Check sheet for the drawn part. Datum: minimum x, y, z corner. Units: mm. A direction names the side the tool comes from. Round coordinates to 2 decimals unless told otherwise and drop trailing zeros. Write each loop counter-clockwise with the first axis right and the second up, starting at its lowest first coordinate (ties: lowest second). Pieces come first, ordered by that corner, then holes. Notation, with made-up numbers: (-17, 78) - (-6, 78) arc R20 ccw to (-6, 109) - close; hole circle Ø5 at (-3, 36). An arc over 180 degrees is marked (long way). Answer as a JSON object with one key per item and string values. Group by question number.
Item 1: Sectioned sample at D-D on z = 56.5. Record the boundary of the cut face in (x, y), plus the area to 3 significant figures.
Item 2: Release check for a two-part mould opening along Y. For the marked faces 1, 2, 3 and 4 record: pulls with the +Y half, pulls with the -Y half, needs draft (parallel to the pull), parting line crosses it, or undercut.
Item 3: Thickness scan on line 1 (Z direction, x = 70, y = 37.5); line 2 (Z direction, x = 38, y = 93); line 3 (Y direction, x = 38, z = 20). Record the ranges inside material, lowest first.
Item 4: Sectioned sample at B-B on x = 47. Record the boundary of the cut face in (y, z).
Item 5: Sectioned sample at C-C on y = 93.98. Record the boundary of the cut face in (x, z).
Item 6: Gauge pin test, flat ends, axial feed: P1, Ø12, axis at y = 93.98, z = 20.32, coming from the -X side; P2, Ø8, axis at x = 41.5, y = 31.5, coming from the +Z side; P3, Ø1.5, axis at x = 60.5, y = 121, coming from the -Z side. Record the tip position at first contact, or that the pin passes through.
Item 7: Set-up check for the marked faces 5 and 6: record each of +Z, -Z, +X, -X, +Y, -Y from which the full face is reachable in a straight line by a thin tool's end or side.
Item 8: Sectioned sample at A-A on z = 20.32. Record the boundary of the cut face in (x, y).
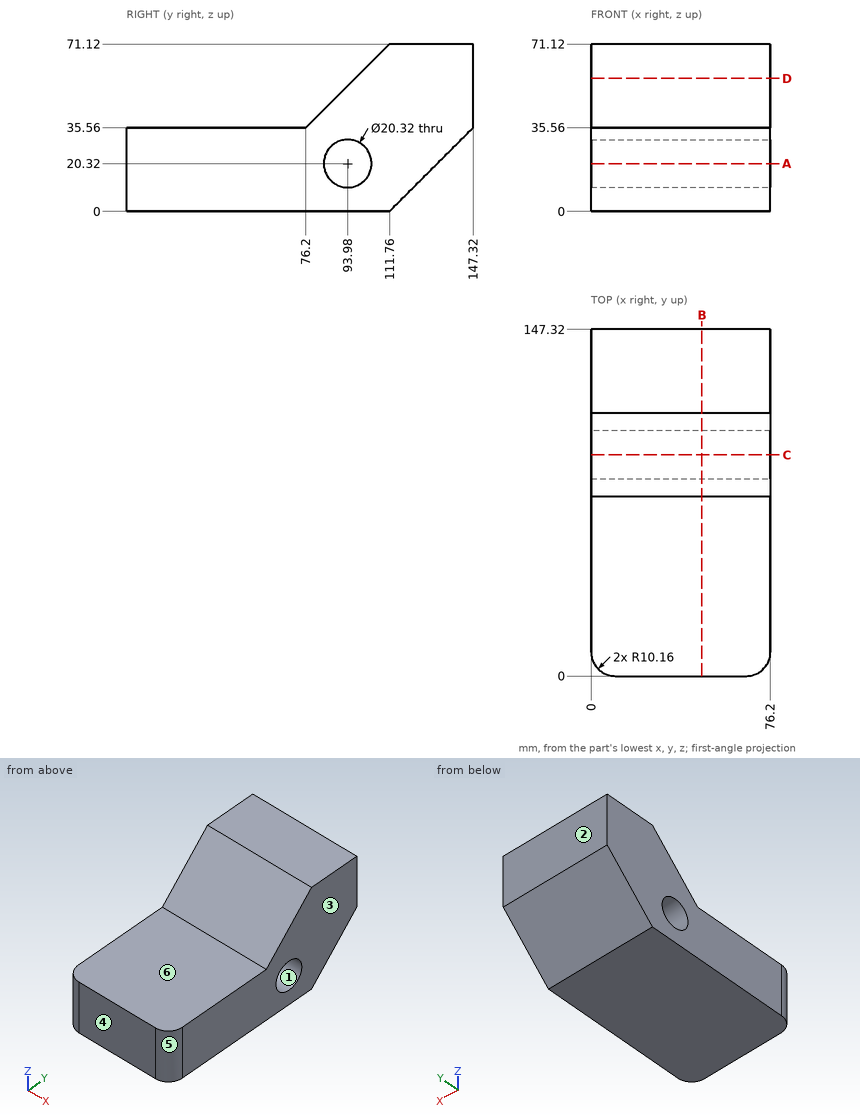
Completed:
{
 "1": {"outline": "(0, 97.14) - (76.2, 97.14) - (76.2, 147.32) - (0, 147.32) - close", "area": "3,820 mm²"},
 "2": {"face 1": "undercut", "face 2": "pulls with the +Y half", "face 3": "needs draft", "face 4": "pulls with the -Y half"},
 "3": {"line 1": "0 to 35.56", "line 2": "0 to 10.21, 30.43 to 52.36", "line 3": "0 to 83.83, 104.13 to 131.76"},
 "4": {"outline": "(0, 0) - (111.76, 0) - (147.32, 35.56) - (147.32, 71.12) - (111.76, 71.12) - (76.2, 35.56) - (0, 35.56) - close; hole circle Ø20.32 at (93.98, 20.32)"},
 "5": {"outline": "(0, 0) - (76.2, 0) - (76.2, 10.16) - (0, 10.16) - close; (0, 30.48) - (76.2, 30.48) - (76.2, 53.34) - (0, 53.34) - close"},
 "6": {"P1": "through", "P2": "z = 35.56", "P3": "z = 8.49"},
 "7": {"face 5": "+Z, -Z, +X, -Y", "face 6": "+Z, +X, -X, -Y"},
 "8": {"outline": "(0, 10.16) arc R10.16 ccw to (10.16, 0) - (66.04, 0) arc R10.16 ccw to (76.2, 10.16) - (76.2, 83.82) - (0, 83.82) - close; (0, 104.14) - (76.2, 104.14) - (76.2, 132.08) - (0, 132.08) - close"}
}
